The figure shows three views and two pictorial views of one solid part (mm, origin at its lowest corner). Answer the questions. A direction names the side the tool comes from. Give positions to 0.01 mm unless a question says otherwise; leave off trailing zeros. Loops run counter-clockwise (first coordinate to the right, second up) from the corner with the lowest first, then second, coordinate; pieces in that order, holes last. Notation, with made-up numbers: (67.5, 59) - (96.5, 59) arc R22 ccw to (96.5, 80) - close; hole circle Ø4 at (56.5, 79). An arc over 180 degrees is marked (long way). Write each question's results on one line, items separated by ' | '.
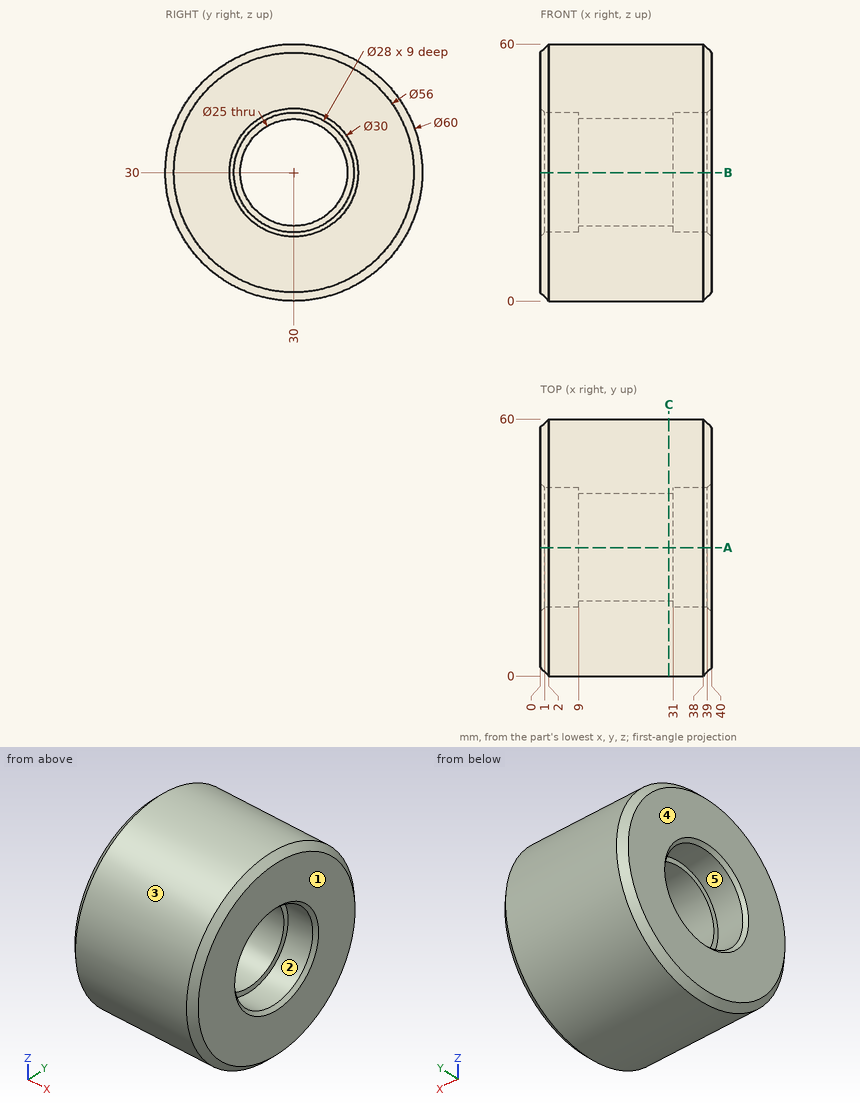
Item 1: A cutting plane is placed at A-A, the plane y = 30. Determine the outline of the cut face in (x, z), plus the area to 3 significant figures.
Values found:
outline: (0, 2) - (2, 0) - (38, 0) - (40, 2) - (40, 15) - (39, 16) - (31, 16) - (31, 17.5) - (9, 17.5) - (9, 16) - (1, 16) - (0, 15) - close; (0, 45) - (1, 44) - (9, 44) - (9, 42.5) - (31, 42.5) - (31, 44) - (39, 44) - (40, 45) - (40, 58) - (38, 60) - (2, 60) - (0, 58) - close | area: 1,340 mm²
Item 2: Find the intervals of material crossed by line 1 along Y through (x, z) = (18, 30); line 2 along Y through (x, z) = (6.25, 30); line 3 along Z through (x, y) = (8, 34), in increasing order. Write a range as [from, to].
Values found:
line 1: y = [0, 17.5], [42.5, 60] | line 2: y = [0, 16], [44, 60] | line 3: z = [0.27, 16.58], [43.42, 59.73]
Item 3: A cutting plane is placed at C-C, the plane x = 30. Determine the outline of the cut face in (y, z), plus the area to 3 significant figures.
Values found:
outline: circle Ø60 at (30, 30); hole circle Ø25 at (30, 30) | area: 2,340 mm²
Item 4: Flat-ended cylindrical pins translate along their axes: P1, Ø17, axis at y = 30, z = 30, coming from the +X side; P2, Ø1.5, axis at x = 32.5, z = 16, coming from the +Y side; P3, Ø1, axis at x = 33.5, z = 16.5, coming from the -Y side; P4, Ø6, axis at x = 10.5, z = 14, coming from the +Y side. Find the tip coordinate at first contact, or state that the pin passes through.
Values found:
P1: passes through | P2: stops at y = 56.92 | P3: stops at y = 2.96 | P4: stops at y = 57.04
Item 5: For the marked faces 1 and 2, determine the directions among +Z, -Z, +X, -X, +Y, -Y from which every point of the face is accessible in a straight line to the end or side of a thin tool.
Values found:
face 1: +Z, -Z, +X, +Y, -Y | face 2: +X
Item 6: For a pull along Z with two mould halves and no side action, classify the marked faces 3, 4 and 5 as released by +Z, released by -Z, zero draft, split by the parting line, or undercut.
Values found:
face 3: split by the parting line | face 4: zero draft | face 5: undercut
